```python
from build123d import *

# Parameters (mm, degrees)
SKETCH1_W           = 155.4
SKETCH1_H           = 86.98
SKETCH1_W_2         = 146
SKETCH1_H_2         = 77.58
BOSS_EXTRUDE2_DEPTH = 1.5
SKETCH1_4_W         = 155.4
SKETCH1_4_H         = 86.98
SKETCH1_4_W_2       = 152.4
SKETCH1_4_H_2       = 83.98
BOSS_EXTRUDE3_DEPTH = 15
FILLET1_R           = 2
FILLET2_R           = 1
FILLET3_R           = 1
BOSS_EXTRUDE4_DEPTH = 0.8
BOSS_EXTRUDE5_DEPTH = 1
BOSS_EXTRUDE6_DEPTH = 1.5


with BuildPart() as part:
    # Sketch1 → Boss-Extrude2 (new body)
    with BuildSketch(Plane(origin=(0, 0, -28.222648695), x_dir=(-1, 0, 0), z_dir=(0, 0, -1))):
        with Locations((-64.074179317, 56.745922466)):
            Rectangle(SKETCH1_W, SKETCH1_H)
        with Locations((-64.074179317, 56.745922466)):
            Rectangle(SKETCH1_W_2, SKETCH1_H_2, mode=Mode.SUBTRACT)
    extrude(amount=BOSS_EXTRUDE2_DEPTH)

    # Sketch1_4 → Boss-Extrude3 (add)
    with BuildSketch(Plane(origin=(0, 0, -28.222648695), x_dir=(-1, 0, 0), z_dir=(0, 0, -1))):
        with Locations((-64.074179317, 56.745922466)):
            Rectangle(SKETCH1_4_W, SKETCH1_4_H)
        with Locations((-64.074179317, 56.745922466)):
            Rectangle(SKETCH1_4_W_2, SKETCH1_4_H_2, mode=Mode.SUBTRACT)
    extrude(amount=-BOSS_EXTRUDE3_DEPTH)

    # Fillet1
    fillet1_edges = [part.edges().sort_by_distance(p)[0] for p in [
        (141.774179317, 100.235922466, -21.472648695),
        (-13.625820683, 100.235922466, -21.472648695),
        (-13.625820683, 13.255922466, -21.472648695),
        (141.774179317, 13.255922466, -21.472648695),
    ]]
    fillet(fillet1_edges, radius=FILLET1_R)

    # Fillet2
    fillet2_edges = [part.edges().sort_by_distance(p)[0] for p in [
        (137.074179317, 17.955922466, -28.972648695),
        (-8.925820683, 17.955922466, -28.972648695),
        (-8.925820683, 95.535922466, -28.972648695),
        (137.074179317, 95.535922466, -28.972648695),
        (137.074179317, 56.745922466, -29.722648695),
        (64.074179317, 95.535922466, -29.722648695),
        (-8.925820683, 56.745922466, -29.722648695),
        (64.074179317, 17.955922466, -29.722648695),
        (141.774179317, 56.745922466, -29.722648695),
        (64.074179317, 100.235922466, -29.722648695),
        (64.074179317, 13.255922466, -29.722648695),
        (-13.625820683, 56.745922466, -29.722648695),
        (141.188392879, 13.841708903, -29.722648695),
        (-13.040034245, 13.841708903, -29.722648695),
        (-13.040034245, 99.650136028, -29.722648695),
        (141.188392879, 99.650136028, -29.722648695),
    ]]
    fillet(fillet2_edges, radius=FILLET2_R)

    # Fillet3
    fillet3_edges = [part.edges().sort_by_distance(p)[0] for p in [
        (141.774179317, 56.745922466, -13.222648695),
        (64.074179317, 100.235922466, -13.222648695),
        (-13.625820683, 56.745922466, -13.222648695),
        (64.074179317, 13.255922466, -13.222648695),
        (141.188392879, 13.841708903, -13.222648695),
        (-13.040034245, 13.841708903, -13.222648695),
        (-13.040034245, 99.650136028, -13.222648695),
        (141.188392879, 99.650136028, -13.222648695),
    ]]
    fillet(fillet3_edges, radius=FILLET3_R)

    # Sketch2 → Boss-Extrude4 (add)
    with BuildSketch(Plane(origin=(0, 14.755922466, 0), x_dir=(1, 0, 0), z_dir=(0, 1, 0))):
        with BuildLine():
            Line((-2.675820683, 22.595795996), (-6.175820683, 22.595795996))
            ThreePointArc((-6.175820683, 22.595795996), (-5.538109989, 18.139864796), (-1.750820683, 20.572648695))
            ThreePointArc((-1.750820683, 20.572648695), (-1.993036784, 21.684938001), (-2.675820683, 22.595795996))
        make_face()
        with BuildLine():
            Line((106.324179317, 22.595795996), (102.824179317, 22.595795996))
            ThreePointArc((102.824179317, 22.595795996), (103.461890011, 18.139864796), (107.249179317, 20.572648695))
            ThreePointArc((107.249179317, 20.572648695), (107.006963216, 21.684938001), (106.324179317, 22.595795996))
        make_face()
    extrude(amount=BOSS_EXTRUDE4_DEPTH)

    # Sketch4 → Boss-Extrude5 (add)
    with BuildSketch(Plane.XZ.offset(-98.735922466)):
        with BuildLine():
            ThreePointArc((135.249179317, -20.572648695), (131.461890011, -18.139864796), (130.824179317, -22.595795996))
            Line((130.824179317, -22.595795996), (134.324179317, -22.595795996))
            ThreePointArc((134.324179317, -22.595795996), (135.006963216, -21.684938001), (135.249179317, -20.572648695))
        make_face()
        with BuildLine():
            ThreePointArc((-1.750820683, -20.572648695), (-5.538109989, -18.139864796), (-6.175820683, -22.595795996))
            Line((-6.175820683, -22.595795996), (-2.675820683, -22.595795996))
            ThreePointArc((-2.675820683, -22.595795996), (-1.993036784, -21.684938001), (-1.750820683, -20.572648695))
        make_face()
    extrude(amount=BOSS_EXTRUDE5_DEPTH)

    # Sketch2_3 → Boss-Extrude6 (add)
    with BuildSketch(Plane(origin=(0, 14.755922466, 0), x_dir=(1, 0, 0), z_dir=(0, 1, 0))):
        with BuildLine():
            Line((106.324179317, 22.595795996), (102.824179317, 22.595795996))
            ThreePointArc((102.824179317, 22.595795996), (103.461890011, 18.139864796), (107.249179317, 20.572648695))
            ThreePointArc((107.249179317, 20.572648695), (107.006963216, 21.684938001), (106.324179317, 22.595795996))
        make_face()
    extrude(amount=BOSS_EXTRUDE6_DEPTH)


solid = part.part
```
Model file for the job. Use its own axes, mm. A direction names the side the tool comes from. Round coordinates to 2 decimals unless told otherwise and drop trailing zeros. Order: outer loops, then holes, each group sorted by start corner. A loop starts at its lowest first (then second) coordinate and runs counter-clockwise, first axis right, second up. Notation, with made-up numbers: (67, 89) -> (104, 89) arc R26 cw to (104, 119) -> close; hole circle Ø11 at (20.25, 74). An arc over 180 degrees is marked (long way). Use one line per item in the form item = value.
Item 1: Tool access for faces 1 (the face through (141.774, 56, -22)), 2 (the face through (104.5, 15.5, -17.9)), 3 (the face through (-12.126, 56, -21)): list every direction of +Z, -Z, +X, -X, +Y, -Y with a clear straight run to the whole face (end or side of a thin tool).
Returned:
face_1 = +Z, -Z, +X, +Y, -Y
face_2 = none
face_3 = +Z
Item 2: Cut at C-C, the plane z = -26.75. Write the cut outline in (x, y).
Returned:
outline = (-13.63, 15.26) arc R2 ccw to (-11.63, 13.26) -> (139.77, 13.26) arc R2 ccw to (141.77, 15.26) -> (141.77, 98.24) arc R2 ccw to (139.77, 100.24) -> (-11.63, 100.24) arc R2 ccw to (-13.63, 98.24) -> close; hole (-12.13, 14.76) -> (140.27, 14.76) -> (140.27, 98.74) -> (-12.13, 98.74) -> close
Item 3: Cut at B-B, the plane x = 117.5. Write the cut outline in (y, z), and give its area (3 significant figures).
Returned:
outline = (13.26, -28.72) arc R1 ccw to (14.26, -29.72) -> (16.96, -29.72) arc R1 ccw to (17.96, -28.72) -> (17.96, -28.22) -> (14.76, -28.22) -> (14.76, -13.22) -> (14.26, -13.22) arc R1 ccw to (13.26, -14.22) -> close; (95.54, -28.72) arc R1 ccw to (96.54, -29.72) -> (99.24, -29.72) arc R1 ccw to (100.24, -28.72) -> (100.24, -14.22) arc R1 ccw to (99.24, -13.22) -> (98.74, -13.22) -> (98.74, -28.22) -> (95.54, -28.22) -> close
area = 57.8 mm^2
Item 4: Pull direction Y, two halves, no side cores. Call faces 4 (the face through (65, 13.256, -22)), 5 (the face through (-13.626, 56, -22)), 6 (the face through (140.274, 56, -21)), 7 (the face through (65, 100.236, -22)): released by +Y, released by -Y, zero draft, split by the parting line, or undercut.
Returned:
face_4 = released by -Y
face_5 = zero draft
face_6 = undercut
face_7 = released by +Y
Item 5: Drill centre lines: line 1 (Y direction, x = 64, z = -25.75); line 2 (X direction, y = 60, z = -28.75); line 3 (X direction, y = 59, z = -19.25). Where is each one in solid material? Low to high.
Returned:
line_1 = 13.26 to 14.76, 98.74 to 100.24
line_2 = -13.63 to -8.93, 137.07 to 141.77
line_3 = -13.63 to -12.13, 140.27 to 141.77
Item 6: Cut at A-A, the plane y = 60. Write the cut outline in (x, z).
Returned:
outline = (-13.63, -28.72) arc R1 ccw to (-12.63, -29.72) -> (-9.93, -29.72) arc R1 ccw to (-8.93, -28.72) -> (-8.93, -28.22) -> (-12.13, -28.22) -> (-12.13, -13.22) -> (-12.63, -13.22) arc R1 ccw to (-13.63, -14.22) -> close; (137.07, -28.72) arc R1 ccw to (138.07, -29.72) -> (140.77, -29.72) arc R1 ccw to (141.77, -28.72) -> (141.77, -14.22) arc R1 ccw to (140.77, -13.22) -> (140.27, -13.22) -> (140.27, -28.22) -> (137.07, -28.22) -> close
